The model under review builds one solid part; all positions refer to its coordinate system, in mm. A direction names the side the tool comes from. Round coordinates to 2 decimals unless told otherwise and drop trailing zeros. Write each loop counter-clockwise with the first axis right and the second up, starting at its lowest first coordinate (ties: lowest second). Pieces come first, ordered by that corner, then holes.
Item 1: Draft analysis for pull direction X (two halves, no side actions). For faces 3 (the face through (-112.554, -9, 11)), 4 (the face through (66.59, -9, 90)), 5 (the face through (-105, -9, 94.187)), state which applies: +X half, -X half, draft (parallel to the pull), parting line (faces both ways), or undercut.
Item 2: Add section A-A (y = -13.25). Give the boundary of the cut face in (x, z).
Item 3: Machinability: for faces 1 (the face through (86, -9, 86.187)), 2 (the face through (114, -9, 94.187)), which of the approach directions +Z, -Z, +X, -X, +Y, -Y give a long, thin tool a straight path to every point of the face, cutting with its end or side? Answer none if there is none.
Item 4: To check wall thickness, follow L1, parallel to X at y = -4, z = 87; L2, parallel to Z at x = -70, y = -8. State the ranges of each line that lie inside material, in increasing order.
Item 5: Add section B-B (x = -67.5). Give the boundary of the cut face in (y, z), plus the area to 3 significant figures.
Item 6: Clearance check with a flat-ended pin moving along its axis: pin 1 Ø5.5 at (x, y) = (-81.5, -10.5) entering from +Z. State where the tip first meets the part, or that it passes through.
```python
from build123d import *

# Parameters (mm, degrees)
F0_W     = 235
F0_H     = 165
F1_DEPTH = 18
F2_W     = 40
F2_H     = 18
F3_DEPTH = 8
F4_W     = 40
F4_H     = 18
F5_DEPTH = 8


with BuildPart() as f1:
    # F0 (on Front) → F1 (new body)
    with BuildSketch(Plane.XZ):
        with Locations((4.946282, 11.687499)):
            Rectangle(F0_W, F0_H)
    extrude(amount=F1_DEPTH)

    # F2 (on face) → F3 (cut)
    with BuildSketch(Plane.XY.offset(94.187499)):
        with Locations((86.589683, -9)):
            Rectangle(F2_W, F2_H)
    extrude(amount=-F3_DEPTH, mode=Mode.SUBTRACT)

    # F4 (on face) → F5 (cut)
    with BuildSketch(Plane.XY.offset(94.187499)):
        with Locations((-76.956588, -9)):
            Rectangle(F4_W, F4_H)
    extrude(amount=-F5_DEPTH, mode=Mode.SUBTRACT)


solid = f1.part
```
Numbers:
1. face 3: -X half
1. face 4: undercut
1. face 5: draft
2. outline: (-112.55, -70.81) - (122.45, -70.81) - (122.45, 94.19) - (106.59, 94.19) - (106.59, 86.19) - (66.59, 86.19) - (66.59, 94.19) - (-56.96, 94.19) - (-56.96, 86.19) - (-96.96, 86.19) - (-96.96, 94.19) - (-112.55, 94.19) - close
3. face 1: +Z, +Y, -Y
3. face 2: +Z, +X, -X, +Y, -Y
4. L1: x = -112.55 to -96.96, -56.96 to 66.59, 106.59 to 122.45
4. L2: z = -70.81 to 86.19
5. outline: (-18, -70.81) - (0, -70.81) - (0, 86.19) - (-18, 86.19) - close
5. area: 2,830 mm2
6. pin 1: stops at z = 86.19
